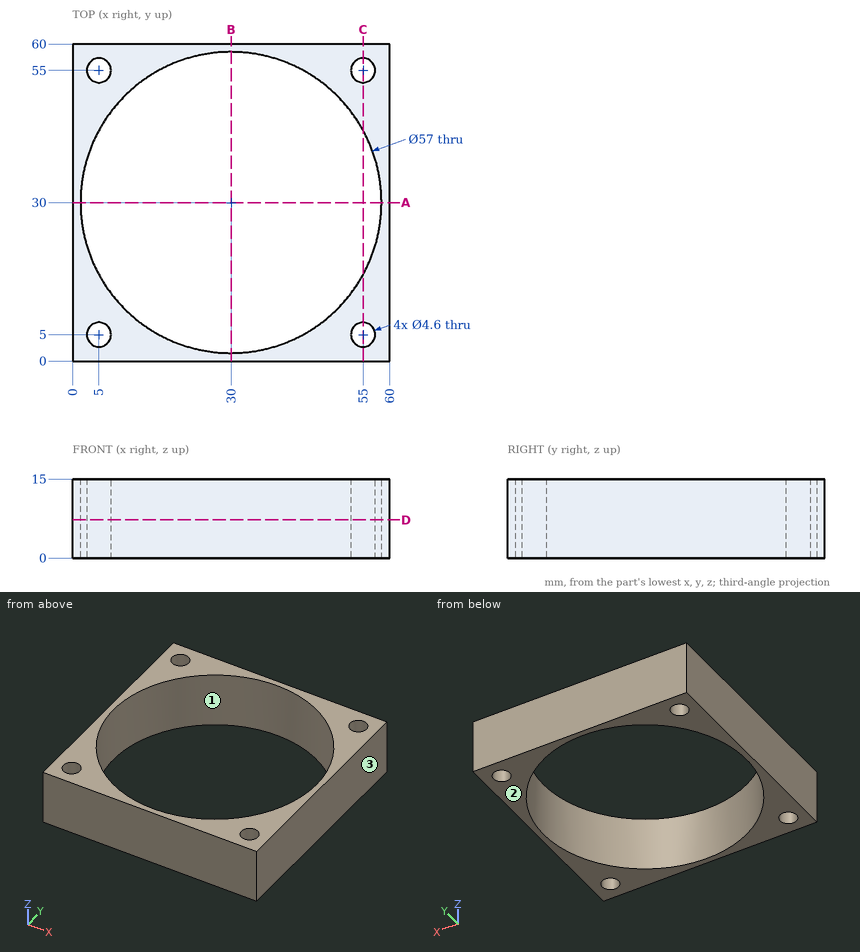
Print and shaded views of the part. All mm, measured from the part's lowest x, y and z. Give positions to 0.01 mm unless a question says otherwise; leave off trailing zeros. Loops run counter-clockwise (first coordinate to the right, second up) from the corner with the lowest first, then second, coordinate; pieces in that order, holes last. Notation, with made-up numbers: (1.25, 74) -> (51.25, 74) arc R37 cw to (51.25, 110) -> close; hole circle Ø6 at (39.5, 6). An arc over 180 degrees is marked (long way). Use a Markdown table: item, result.
1. Flat gauge pin, fed straight in: pin 1 (3.5 mm diameter, centred on x = 5, y = 55, fed in from -Z). Where does the tip first touch, or does it go through?
Check result:
| item | result |
|---|---|
| pin 1 | passes through |
2. Slice it at A-A (y = 30). List the corners of the cut face in (x, z).
Check result:
| item | result |
|---|---|
| outline | (0, 0) -> (1.5, 0) -> (1.5, 15) -> (0, 15) -> close; (58.5, 0) -> (60, 0) -> (60, 15) -> (58.5, 15) -> close |
3. Slice it at D-D (z = 7.25). List the corners of the cut face in (x, y).
Check result:
| item | result |
|---|---|
| outline | (0, 0) -> (60, 0) -> (60, 60) -> (0, 60) -> close; hole circle Ø57 at (30, 30); hole circle Ø4.6 at (5, 5); hole circle Ø4.6 at (5, 55); hole circle Ø4.6 at (55, 5); hole circle Ø4.6 at (55, 55) |
4. Slice it at C-C (x = 55). List the corners of the cut face in (y, z).
Check result:
| item | result |
|---|---|
| outline | (0, 0) -> (2.7, 0) -> (2.7, 15) -> (0, 15) -> close; (7.3, 0) -> (16.32, 0) -> (16.32, 15) -> (7.3, 15) -> close; (43.68, 0) -> (52.7, 0) -> (52.7, 15) -> (43.68, 15) -> close; (57.3, 0) -> (60, 0) -> (60, 15) -> (57.3, 15) -> close |
5. Mould opens along X. For the marked faces 1, 2 and 3 say: pulls with the +X half, pulls with the -X half, needs draft (parallel to the pull), parting line crosses it, or undercut.
Check result:
| item | result |
|---|---|
| face 1 | undercut |
| face 2 | needs draft |
| face 3 | pulls with the +X half |
6. Wall check: L1, parallel to Y at x = 30, z = 8.75; L2, parallel to Y at x = 55, z = 6.75; L3, parallel to X at y = 54.5, z = 2 (3 decimals). Give the ranges that are in metal, low to high. Write a range as [from, to].
Check result:
| item | result |
|---|---|
| L1 | y = [0, 1.5], [58.5, 60] |
| L2 | y = [0, 2.7], [7.3, 16.32], [43.68, 52.7], [57.3, 60] |
| L3 | x = [0, 2.755], [7.245, 15.44], [44.56, 52.755], [57.245, 60] |
